```python
from build123d import *

# Parameters (mm, degrees)
SKETCH1_W           = 20
SKETCH1_H           = 20
BOSS_EXTRUDE1_DEPTH = 2
SKETCH2_R           = 9.75
SKETCH2_R_2         = 8.75
BOSS_EXTRUDE2_DEPTH = 6
BOSS_EXTRUDE3_DEPTH = 9
CUT_EXTRUDE4_DEPTH  = 6
SKETCH6_R           = 0.875
CUT_EXTRUDE5_DEPTH  = 6
BOSS_EXTRUDE4_DEPTH = 1
SKETCH8_R           = 0.6
CUT_EXTRUDE6_DEPTH  = 12


with BuildPart() as part:
    # Sketch1 → Boss-Extrude1 (new body)
    with BuildSketch(Plane(origin=(0, 0, 0), x_dir=(1, 0, 0), z_dir=(0, 1, 0))):
        with Locations((-25.908439561, -86.922355933)):
            Rectangle(SKETCH1_W, SKETCH1_H)
    extrude(amount=BOSS_EXTRUDE1_DEPTH)

    # Sketch2 → Boss-Extrude2 (add)
    with BuildSketch(Plane(origin=(0, 2, 0), x_dir=(1, 0, 0), z_dir=(0, 1, 0))):
        with Locations(Location((-25.908439561, -86.922355933, 0), (0, 0, 90))):
            Circle(SKETCH2_R)
        with Locations(Location((-25.908439561, -86.922355933, 0), (0, 0, 270))):
            Circle(SKETCH2_R_2, mode=Mode.SUBTRACT)
    extrude(amount=BOSS_EXTRUDE2_DEPTH)

    # Sketch3 → Boss-Extrude3 (add)
    with BuildSketch(Plane(origin=(0, 2, 0), x_dir=(1, 0, 0), z_dir=(0, 1, 0))):
        with BuildLine():
            Line((-27.877576428, -86.572355933), (-25.908439561, -86.572355933))
            Line((-25.908439561, -86.572355933), (-23.939302694, -86.572355933))
            ThreePointArc((-23.939302694, -86.572355933), (-25.908439561, -84.922355933), (-27.877576428, -86.572355933))
        make_face()
        with BuildLine():
            Line((-23.939302694, -87.272355933), (-27.877576428, -87.272355933))
            ThreePointArc((-27.877576428, -87.272355933), (-25.908439561, -88.922355933), (-23.939302694, -87.272355933))
        make_face()
    extrude(amount=BOSS_EXTRUDE3_DEPTH)

    # Sketch4 → Cut-Extrude4 (cut)
    with BuildSketch(Plane.XY.offset(86.572355933)):
        Polygon((-25.033439561, 10.95), (-26.783439561, 10.95), (-26.783439561, 9.2), (-25.908439561, 9.2), (-25.033439561, 9.2), align=None)
    extrude(amount=-CUT_EXTRUDE4_DEPTH, mode=Mode.SUBTRACT)

    # Sketch6 → Cut-Extrude5 (cut)
    with BuildSketch(Plane(origin=(0, 0, 87.272355933), x_dir=(-1, 0, 0), z_dir=(0, 0, -1))):
        with Locations((25.908439561, 10.075)):
            Circle(SKETCH6_R)
    extrude(amount=-CUT_EXTRUDE5_DEPTH, mode=Mode.SUBTRACT)

    # Sketch7 → Boss-Extrude4 (add)
    with BuildSketch(Plane(origin=(0, 11, 0), x_dir=(1, 0, 0), z_dir=(0, 1, 0))):
        with BuildLine():
            Line((-27.877576428, -86.572355933), (-23.939302694, -86.572355933))
            ThreePointArc((-23.939302694, -86.572355933), (-25.908439561, -84.922355933), (-27.877576428, -86.572355933))
        make_face()
        with BuildLine():
            Line((-23.939302694, -87.272355933), (-27.877576428, -87.272355933))
            ThreePointArc((-27.877576428, -87.272355933), (-25.908439561, -88.922355933), (-23.939302694, -87.272355933))
        make_face()
    extrude(amount=BOSS_EXTRUDE4_DEPTH)

    # Sketch8 → Cut-Extrude6 (cut)
    with BuildSketch(Plane(origin=(0, 0, 76.922355933), x_dir=(-1, 0, 0), z_dir=(0, 0, -1))):
        with Locations((18.908439561, 5)):
            Circle(SKETCH8_R)
    extrude(amount=-CUT_EXTRUDE6_DEPTH, mode=Mode.SUBTRACT)


solid = part.part
```
Input: part model. Units: mm. Frame: model coordinates. A direction names the side the tool comes from. Round coordinates to 2 decimals unless told otherwise and drop trailing zeros. Loops run counter-clockwise (first coordinate to the right, second up) from the corner with the lowest first, then second, coordinate; pieces in that order, holes last. Notation, with made-up numbers: (-14.75, 85.5) - (-6.75, 85.5) arc R29 ccw to (-6.75, 113.5) - close; hole circle Ø4 at (-33.75, 0.5). An arc over 180 degrees is marked (long way). One line per item, written item: value. Start each with the question number.
(1) Access query for faces 1 (the flat face through (-35.908, 1, 87)), 2 (the cylindrical face through (-18.31, 5.03, 81.06)), 3 (the cylindrical face through (-25.52, 4.96, 78.18)). Directions: +Z, -Z, +X, -X, +Y, -Y. A direction counts if a zero-diameter tool reaches every point of the face in a straight line with its end or side. Return the directions, or none.
(2) Section C-C, the plane y = 5. Return loops of the section in (x, z), plus the area to 3 significant figures.
(3) Ray query, line 1 (Y direction, x = -26.5, z = 92.5); line 2 (X direction, y = 3, z = 85.75); line 3 (Y direction, x = -17, z = 90). Return the intervals inside material, ascending. Write a range as [from, to].
(4) Section D-D, the plane z = 82. Return loops of the section in (x, y).
(5) Section A-A, the plane y = 7.5. Return loops of the section in (x, z), plus the area to 3 significant figures.
(6) Section B-B, the plane x = -19. Return loops of the section in (y, z), plus the area to 3 significant figures.
(7) Contact query for flat-ended pins moving along their axis: P1, Ø4, axis at y = 6.5, z = 82.5, coming from the +X side; P2, Ø0.5, axis at x = -26, z = 85.5, coming from the -Y side; P3, Ø3, axis at x = -26, y = 8.5, coming from the -Z side; P4, Ø1.2, axis at y = 10, z = 85.5, coming from the +X side. Output: stop coordinate, or through.
(8) Draft query along Z for faces 4 (the flat face through (-26, 1, 76.922)), 5 (the flat face through (-26, 12, 86)), 6 (the cylindrical face through (-25.95, 6.93, 88.92)). Return one class per face: +Z half, -Z half, draft (parallel to the pull), parting line (faces both ways), or undercut.
Results below:
1. face 1: +Z, -Z, -X, +Y, -Y
1. face 2: -Z
1. face 3: +Y
2. outline: (-27.88, 86.57) arc R2 ccw to (-23.94, 86.57) - close; (-27.88, 87.27) - (-23.94, 87.27) arc R2 ccw to start; (-19.51, 79.57) - (-19.51, 80.96) arc R8.75 cw (long way) to (-18.31, 82.59) - (-18.31, 80.81) arc R9.75 ccw (long way) to start
2. area: 66.0 mm^2
3. line 1: [0, 2]
3. line 2: [-35.59, -34.58], [-27.53, -24.29], [-17.24, -16.23]
3. line 3: [0, 8]
4. outline: (-35.91, 0) - (-15.91, 0) - (-15.91, 2) - (-17.49, 2) - (-17.49, 8) - (-18.67, 8) - (-18.67, 5.55) arc R0.6 cw to (-18.67, 4.45) - (-18.67, 2) - (-33.14, 2) - (-33.14, 8) - (-34.32, 8) - (-34.32, 2) - (-35.91, 2) - close
5. outline: circle Ø19.5 at (-25.91, 86.92); (-27.88, 86.57) arc R2 ccw to (-23.94, 86.57) - close; (-27.88, 87.27) - (-23.94, 87.27) arc R2 ccw to start; hole circle Ø17.5 at (-25.91, 86.92)
5. area: 67.9 mm^2
6. outline: (0, 76.92) - (2, 76.92) - (2, 80.04) - (4.41, 80.04) - (4.41, 81.55) - (2, 81.55) - (2, 92.29) - (8, 92.29) - (8, 93.8) - (2, 93.8) - (2, 96.92) - (0, 96.92) - close; (5.59, 80.04) - (8, 80.04) - (8, 81.55) - (5.59, 81.55) - close
6. area: 56.3 mm^2
7. P1: x = -16.46
7. P2: y = 0
7. P3: z = 77.17
7. P4: x = -24.09
8. face 4: -Z half
8. face 5: draft
8. face 6: undercut
